from build123d import *

# Parameters (mm, degrees)
F1_DEPTH = 5
F2_DEPTH = 30
F3_R     = 10
F4_DEPTH = 40


with BuildPart() as f1:
    # F0 (on Front) → F1 (new body)
    with BuildSketch(Plane.XZ):
        with BuildLine():
            Line((17.5, -7.5), (32.5, -7.5))
            Line((32.5, -7.5), (32.5, 7.5))
            Line((32.5, 7.5), (17.5, 7.5))
            ThreePointArc((17.5, 7.5), (22.803301, 5.303301), (25, 0))
            ThreePointArc((25, 0), (22.803301, -5.303301), (17.5, -7.5))
        make_face()
        with BuildLine():
            Line((0, -7.5), (17.5, -7.5))
            ThreePointArc((17.5, -7.5), (12.196699, -5.303301), (10, 0))
            Line((10, 0), (7.5, 0))
            ThreePointArc((7.5, 0), (5.303301, -5.303301), (0, -7.5))
        make_face()
        with BuildLine():
            ThreePointArc((10, 0), (12.196699, -5.303301), (17.5, -7.5))
            ThreePointArc((17.5, -7.5), (22.803301, -5.303301), (25, 0))
            ThreePointArc((25, 0), (22.803301, 5.303301), (17.5, 7.5))
            ThreePointArc((17.5, 7.5), (12.196699, 5.303301), (10, 0))
        make_face()
        with BuildLine():
            Line((-17.5, -7.5), (0, -7.5))
            ThreePointArc((0, -7.5), (-5.303301, -5.303301), (-7.5, 0))
            Line((-7.5, 0), (-10, 0))
            ThreePointArc((-10, 0), (-12.196699, -5.303301), (-17.5, -7.5))
        make_face()
        with BuildLine():
            Line((7.5, 0), (10, 0))
            ThreePointArc((10, 0), (12.196699, 5.303301), (17.5, 7.5))
            Line((17.5, 7.5), (0, 7.5))
            ThreePointArc((0, 7.5), (5.303301, 5.303301), (7.5, 0))
        make_face()
        with BuildLine():
            Line((-32.5, -7.5), (-17.5, -7.5))
            ThreePointArc((-17.5, -7.5), (-25, 0), (-17.5, 7.5))
            Line((-17.5, 7.5), (-32.5, 7.5))
            Line((-32.5, 7.5), (-32.5, -7.5))
        make_face()
        with BuildLine():
            ThreePointArc((-17.5, 7.5), (-25, 0), (-17.5, -7.5))
            ThreePointArc((-17.5, -7.5), (-12.196699, -5.303301), (-10, 0))
            ThreePointArc((-10, 0), (-12.196699, 5.303301), (-17.5, 7.5))
        make_face()
        with BuildLine():
            Line((-10, 0), (-7.5, 0))
            ThreePointArc((-7.5, 0), (-5.303301, 5.303301), (0, 7.5))
            Line((0, 7.5), (-17.5, 7.5))
            ThreePointArc((-17.5, 7.5), (-12.196699, 5.303301), (-10, 0))
        make_face()
    extrude(amount=F1_DEPTH)

    # F0 (on Front) → F2 (join)
    with BuildSketch(Plane.XZ):
        with BuildLine():
            ThreePointArc((-17.5, 7.5), (-25, 0), (-17.5, -7.5))
            ThreePointArc((-17.5, -7.5), (-12.196699, -5.303301), (-10, 0))
            ThreePointArc((-10, 0), (-12.196699, 5.303301), (-17.5, 7.5))
        make_face()
        with BuildLine():
            ThreePointArc((-7.5, 0), (-5.303301, -5.303301), (0, -7.5))
            ThreePointArc((0, -7.5), (5.303301, -5.303301), (7.5, 0))
            ThreePointArc((7.5, 0), (5.303301, 5.303301), (0, 7.5))
            ThreePointArc((0, 7.5), (-5.303301, 5.303301), (-7.5, 0))
        make_face()
        with BuildLine():
            ThreePointArc((10, 0), (12.196699, -5.303301), (17.5, -7.5))
            ThreePointArc((17.5, -7.5), (22.803301, -5.303301), (25, 0))
            ThreePointArc((25, 0), (22.803301, 5.303301), (17.5, 7.5))
            ThreePointArc((17.5, 7.5), (12.196699, 5.303301), (10, 0))
        make_face()
    extrude(amount=F2_DEPTH)

    # F3 (on Front) → F4 (join)
    with BuildSketch(Plane.XZ):
        Circle(F3_R)
    extrude(amount=-F4_DEPTH)


solid = f1.part
Could you check a few things on this model? Use its own coordinates, in mm. A direction names the side the tool comes from. Coordinates: 2 decimals unless noted, no trailing zeros. Write each loop counter-clockwise with the first axis right and the second up, starting at its lowest first coordinate (ties: lowest second). Pieces come first, ordered by that corner, then holes. Notation, with made-up numbers: M -18,-21 L 39,-21 A15 ccw 39,7 Z; hole C 32,70.5 d1. An arc over 180 degrees is marked long. One line per question, with ' | ' between items.
1) Imagine slicing it at D-D, the plane y = 19.5. Write out the boundary of the cut face in (x, z).
Checks:
outline: C 0,0 d20
2) For pin 1 Ø3 at (y, z) = (8, 3.5) entering from -X; pin 2 Ø1 at (y, z) = (-16.5, -5.5) entering from +X; pin 3 Ø12 at (x, y) = (-25, -11.5) entering from +Z, each with a flat end and sliding along its axis, tell me the tip position at first contact or that it passes through.
Checks:
pin 1: x = -9.8 | pin 2: x = 23.09 | pin 3: z = 7.35
3) For faces 4 (the face through (-2.17, 19.72, -9.76)), 5 (the face through (28, -5, 0)), 6 (the face through (0, 0, -8)), 7 (the face through (9, -5, 0)), which set-ups out of +Z, -Z, +X, -X, +Y, -Y let a thin tool reach every point of the face, with its end or its side?
Checks:
face 4: +Y | face 5: +X, -Y | face 6: -Z, +X, -X, -Y | face 7: -Y
4) Imagine slicing it at C-C, the plane x = -1. Write out the boundary of the cut face in (y, z).
Checks:
outline: M -30,-7.43 L -5,-7.43 L -5,-7.5 L 0,-7.5 L 0,-9.95 L 40,-9.95 L 40,9.95 L 0,9.95 L 0,7.5 L -5,7.5 L -5,7.43 L -30,7.43 Z
5) I need wall thicknesses on probe 1 along X at (y, z) = (-11, -1.25); probe 2 along Z at (x, y) = (-7.5, 6.5); probe 3 along Y at (x, z) = (-14.5, -5.5). Which ranges of each line are inside material? Lowest first, please. Write a range as [from, to].
Checks:
probe 1: [-24.9, -10.1], [-7.4, 7.4], [10.1, 24.9] | probe 2: [-6.61, 6.61] | probe 3: [-30, 0]
6) Imagine slicing it at A-A, the plane y = -23.5. Write out the boundary of the cut face in (x, z).
Checks:
outline: C -17.5,0 d15; C 0,0 d15; C 17.5,0 d15
7) Imagine slicing it at B-B, the plane z = 6. Write out the boundary of the cut face in (x, y), and give its area (3 significant figures).
Checks:
outline: M -32.5,-5 L -22,-5 L -22,-30 L -13,-30 L -13,-5 L -4.5,-5 L -4.5,-30 L 4.5,-30 L 4.5,-5 L 13,-5 L 13,-30 L 22,-30 L 22,-5 L 32.5,-5 L 32.5,0 L 8,0 L 8,40 L -8,40 L -8,0 L -32.5,0 Z | area: 1,640 mm²
8) If we mould it in two halves opening along X, with no side actions, what happens to faces 1 (the face through (-9, -5, 0)), 2 (the face through (32.5, -2, 0)), 3 (the face through (0, 40, 0))? For each: released by +X, released by -X, zero draft, split by the parting line, or undercut.
Checks:
face 1: undercut | face 2: released by +X | face 3: zero draft
